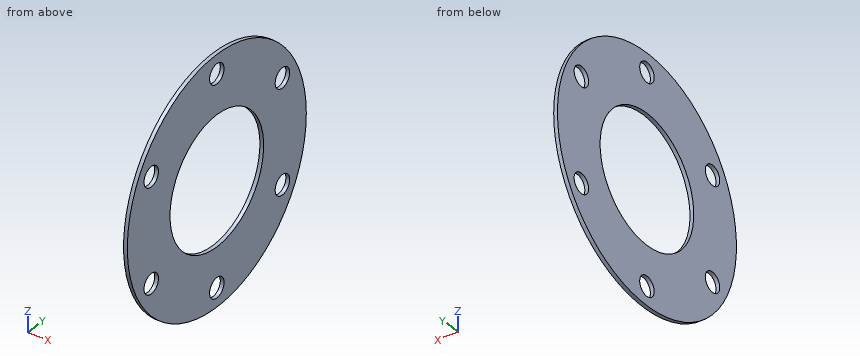
Autodesk Inventor part; units mm, degrees
ref_plane "YZ Plane" through (0, 0, 0) normal (1, 0, 0) x (0, 1, 0)
ref_plane "XZ Plane" through (0, 0, 0) normal (0, 1, 0) x (-1, 0, 0)
ref_plane "XY Plane" through (0, 0, 0) normal (0, 0, 1) x (1, 0, 0)
sketch "Sketch1" plane through (0, 0, 0) normal (1, 0, 0) x (0, 1, 0)
  circle A0 centre (0, 0) radius 65
  dimension "d0" = 130
extrude "Extrusion1" add sketch "Sketch1" along normal blind 2
sketch "Sketch2" plane through (0, 0, 0) normal (-1, 0, 0) x (0, 0, 1)
  circle A0 centre (0, 0) radius 55
  circle A1 centre (-55, 0) radius 5.25
  dimension "d3" = 110
  dimension "d4" = 10.5
hole "Hole1" at (0, 0, -55) direction (1, 0, 0) diameter 10.5 end through all
pattern_circular "Circular Pattern1" count 6 over 360 about axis through (0, 0, 0) along (1, 0, 0) of "Hole1"
sketch "Sketch3" plane through (2, 0, 0) normal (1, 0, 0) x (0, 0, -1)
  circle A0 centre (0, 0) radius 34
  dimension "d15" = 68
extrude "Extrusion2" cut sketch "Sketch3" against normal blind 10
properties part number "04_Dem_dieu_chinh"
The listing builds one solid part. Answer for the finished solid, in the listing's coordinates (mm). Coordinates: 2 decimals unless noted, no trailing zeros. Write each loop counter-clockwise with the first axis right and the second up, starting at its lowest first coordinate (ties: lowest second). Pieces come first, ordered by that corner, then holes. Notation, with made-up numbers: (53.25, 35.5) - (89.25, 35.5) arc R28 ccw to (89.25, 57.5) - close; hole circle Ø5 at (87, 85). An arc over 180 degrees is marked (long way). One line per item, written item: value.
1) Find section B-B (y = 0). Give the vertices of the cut face in (x, z), and give its area (3 significant figures).
Geometry check:
outline: (0, -65) - (2, -65) - (2, -60.25) - (0, -60.25) - close; (0, -49.75) - (2, -49.75) - (2, -34) - (0, -34) - close; (0, 34) - (2, 34) - (2, 49.75) - (0, 49.75) - close; (0, 60.25) - (2, 60.25) - (2, 65) - (0, 65) - close
area: 82.0 mm2
2) Find section A-A (z = 0). Give the vertices of the cut face in (x, y), and give its area (3 significant figures).
Geometry check:
outline: (0, -65) - (2, -65) - (2, -34) - (0, -34) - close; (0, 34) - (2, 34) - (2, 65) - (0, 65) - close
area: 124 mm2
3) Consider line 1 along Z through (x, y) = (1.85, 48); line 2 along Z through (x, y) = (0.2, -1.5); line 3 along Y through (x, z) = (0.7, -7). Determine where each line is inside the solid, lowest interval first. Write a range as from..to.
Geometry check:
line 1: z = -43.83..-32.74, -22.26..22.26, 32.74..43.83
line 2: z = -64.98..-60.03, -49.97..-33.97, 33.97..49.97, 60.03..64.98
line 3: y = -64.62..-33.27, 33.27..64.62
4) Find section C-C (z = -31). Give the vertices of the cut face in (x, y).
Geometry check:
outline: (0, -57.13) - (2, -57.13) - (2, -51.54) - (0, -51.54) - close; (0, -43.72) - (2, -43.72) - (2, -13.96) - (0, -13.96) - close; (0, 13.96) - (2, 13.96) - (2, 43.72) - (0, 43.72) - close; (0, 51.54) - (2, 51.54) - (2, 57.13) - (0, 57.13) - close
5) Find section D-D (x = 0.65). Give the vertices of the cut face in (y, z) (3 decimals).
Geometry check:
outline: circle Ø130 at (0, 0); hole circle Ø10.5 at (-47.631, -27.5); hole circle Ø10.5 at (-47.631, 27.5); hole circle Ø68 at (0, 0); hole circle Ø10.5 at (0, -55); hole circle Ø10.5 at (0, 55); hole circle Ø10.5 at (47.631, -27.5); hole circle Ø10.5 at (47.631, 27.5)
